Drawing for the job (mm, zero at the part's lowest x, y, z). Round coordinates to 2 decimals unless told otherwise and drop trailing zeros. Loops run counter-clockwise (first coordinate to the right, second up) from the corner with the lowest first, then second, coordinate; pieces in that order, holes last. Notation, with made-up numbers: M 41,45 L 58,45 A23 cw 58,80 Z; hole C -27.75,37.5 d3. An arc over 180 degrees is marked long. Use a Markdown table: item, result. Add a question column.
Q1. Pin check, flat tip, straight feed: pin 1 (5 mm diameter, centred on x = 42, y = 25, fed in from +Z). Stop position of the tip, or through.
Q2. Cut at A-A (y = 55). Give the cut face in (x, z).
Q3. Cut at D-D (z = 6). State how many separate pieces and enclosed holes the cut face has, plus the area to 3 significant figures.
Q4. Cut at C-C (y = 15). Give the cut face in (x, z), plus the area to 3 significant figures.
Q5. Probe line 1 (Y direction, x = 42, z = 3.25); line 2 (Y direction, x = 165, z = 5.5); line 3 (X direction, y = 14, z = 9). List the from-to ranges inside material, lowest first. Write a range as from..to.
Q6. Cut at B-B (x = 42). Give the cut face in (y, z), plus the area to 3 significant figures.
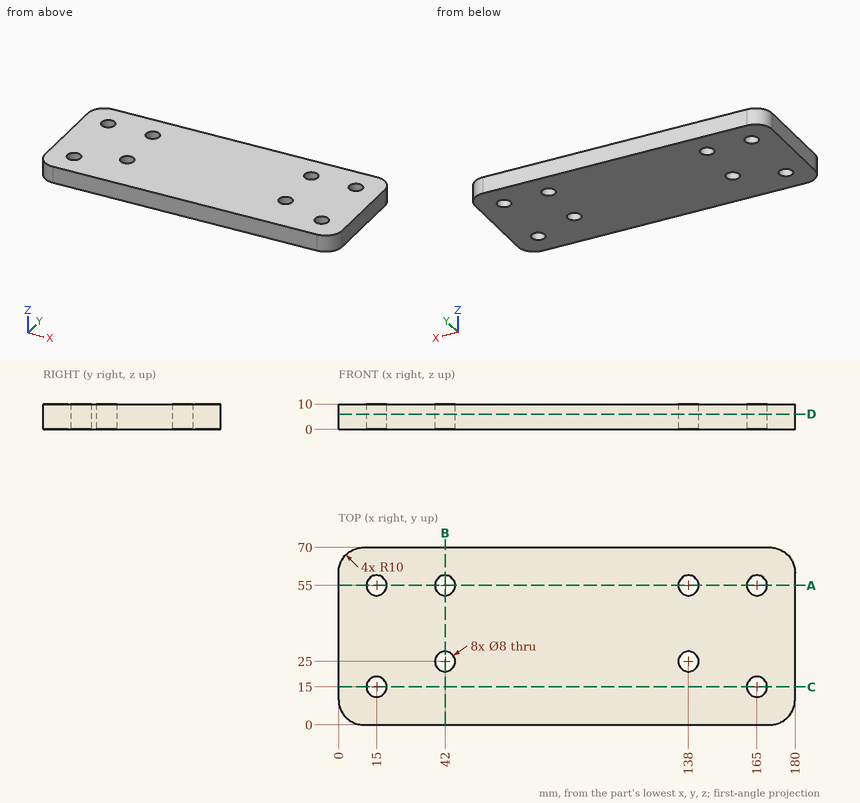
Checked values:
| question | item | result |
|---|---|---|
| 1 | pin 1 | passes through |
| 2 | outline | M 0,0 L 11,0 L 11,10 L 0,10 Z; M 19,0 L 38,0 L 38,10 L 19,10 Z; M 46,0 L 134,0 L 134,10 L 46,10 Z; M 142,0 L 161,0 L 161,10 L 142,10 Z; M 169,0 L 180,0 L 180,10 L 169,10 Z |
| 3 | separate pieces | 1 |
| 3 | enclosed holes | 8 |
| 3 | area | 12,100 mm^2 |
| 4 | outline | M 0,0 L 11,0 L 11,10 L 0,10 Z; M 19,0 L 161,0 L 161,10 L 19,10 Z; M 169,0 L 180,0 L 180,10 L 169,10 Z |
| 4 | area | 1,640 mm^2 |
| 5 | line 1 | y = 0..21, 29..51, 59..70 |
| 5 | line 2 | y = 0..11, 19..51, 59..70 |
| 5 | line 3 | x = 0..11.13, 18.87..161.13, 168.87..180 |
| 6 | outline | M 0,0 L 21,0 L 21,10 L 0,10 Z; M 29,0 L 51,0 L 51,10 L 29,10 Z; M 59,0 L 70,0 L 70,10 L 59,10 Z |
| 6 | area | 540 mm^2 |
